Autodesk Inventor part; units mm, degrees
ref_plane "YZ Plane" through (0, 0, 0) normal (1, 0, 0) x (0, 1, 0)
ref_plane "XZ Plane" through (0, 0, 0) normal (0, 1, 0) x (-1, 0, 0)
ref_plane "XY Plane" through (0, 0, 0) normal (0, 0, 1) x (1, 0, 0)
sketch "Sketch1" plane through (0, 0, 0) normal (0, 0, 1) x (1, 0, 0)
  arc A0 (0, 12.7) -> (0, -12.7) centre (0, 0) ccw
  arc A1 (0, 25.4) -> (0, -25.4) centre (0, 0) ccw
  arc A2 (63.5, -12.7) -> (63.5, 12.7) centre (63.5, 0) ccw
  arc A3 (63.5, -25.4) -> (63.5, 25.4) centre (63.5, 0) ccw
  line L0 (0, 12.7) -> (63.5, 12.7)
  line L1 (0, -12.7) -> (63.5, -12.7)
  line L2 (0, 25.4) -> (63.5, 25.4)
  line L3 (0, -25.4) -> (63.5, -25.4)
  dimension "d0" = 25.4
  dimension "d1" = 50.8
  dimension "d2" = 25.4
  dimension "d3" = 50.8
  dimension "d4" = 63.5
extrude "Extrusion1" add sketch "Sketch1" along normal blind 12.7
sketch "Sketch2" plane through (0, 0, 12.7) normal (0, 0, 1) x (1, 0, 0)
  line L0 (0, -25.4) -> (63.5, -25.4)
  line L1 (31.75, -25.4) -> (31.75, -12.7)
  line L2 (0, -12.7) -> (63.5, -12.7)
  line L3 (47.625, -12.7) -> (47.625, -25.4)
  line L4 (95.25, -31.75) -> (95.25, -25.4)
  line L5 (15.875, -12.7) -> (15.875, -25.4)
  line L6 (15.875, -12.7) -> (47.625, -12.7)
  line L7 (15.875, -25.4) -> (47.625, -25.4)
  point P0 (0, 0)
  dimension "d8" = 15.875
  dimension "d9" = 15.875
extrude "Extrusion2" cut sketch "Sketch2" against normal blind 12.7
sketch "Sketch4" plane through (0, 25.4, 0) normal (0, 1, 0) x (1, 0, 0)
  line L0 (63.5, 0) -> (0, 0)
  circle A0 centre (31.75, -25.4) radius 6.35
  arc A1 (15.875, -25.4) -> (47.625, -25.4) centre (31.75, -25.4) ccw
  line L1 (15.875, -25.4) -> (15.875, -12.7)
  line L2 (0, -12.7) -> (15.875, -12.7)
  line L3 (47.625, -25.4) -> (47.625, -12.7)
  line L4 (0, -12.7) -> (63.5, -12.7)
  line L5 (31.75, 0) -> (31.75, -12.7)
  dimension "d15" = 12.7
  dimension "d16" = 31.75
  dimension "d17" = 25.4
  dimension "d20" = 0
extrude "Extrusion3" add sketch "Sketch4" against normal blind 12.7
properties part number "HW 2 Part 4"
Geometry: final body of the model. Coordinates: model frame, mm. A direction names the side the tool comes from. Coordinates: 2 decimals unless noted, no trailing zeros. Order: outer loops, then holes, each group sorted by start corner. A loop starts at its lowest first (then second) coordinate and runs counter-clockwise, first axis right, second up. Notation, with made-up numbers: (-23, 43) - (-5, 43) arc R30 cw to (-5, 69) - close; hole circle Ø3 at (59, 47.5). An arc over 180 degrees is marked (long way). Write each question's results on one line, items separated by ' | '.
(1) First-contact query: pin 1 Ø14 at (y, z) = (16.5, 19) entering from -X; pin 2 Ø12.5 at (x, y) = (69.5, 3) entering from +Z; pin 3 Ø6.5 at (y, z) = (-18, 8) entering from +X. Flat tips, straight axial feed; report the tip coordinate or a pass-through.
Values found:
pin 1: stops at x = -21.55 | pin 2: stops at z = 12.7 | pin 3: stops at x = 84.18
(2) Mould query, pull axis Y, two halves, no side actions, for faces 1 (the face through (88.894, 0.559, 6.261)), 2 (the face through (-12.697, -0.279, 6.261)), 3 (the face through (47.625, -19, 6)), 4 (the face through (31, 12.7, 16)). Classes: +Y half, -Y half, draft (parallel to the pull), parting line (faces both ways), or undercut.
Values found:
face 1: parting line | face 2: undercut | face 3: draft | face 4: undercut
(3) Section query C-C, the plane z = 10. Return the cut outline in (x, y) (3 decimals), plus the area to 3 significant figures.
Values found:
outline: (0, -25.4) - (15.875, -25.4) - (15.875, -12.7) - (0, -12.7) arc R12.7 cw to (0, 12.7) - (63.5, 12.7) arc R12.7 cw to (63.5, -12.7) - (47.625, -12.7) - (47.625, -25.4) - (63.5, -25.4) arc R25.4 ccw to (63.5, 25.4) - (0, 25.4) arc R25.4 ccw to start | area: 2,730 mm²
(4) Set-up query: faces 5 (the face through (15.875, -19, 6)), 6 (the face through (47.625, 19, 19)), 7 (the face through (55, -12.7, 6)). Return all of +Z, -Z, +X, -X, +Y, -Y with unobstructed straight access to the full face (end or side cutting, diameter ignored); none if empty.
Values found:
face 5: +Z, -Z, -Y | face 6: +Z, +X, +Y, -Y | face 7: +Z, -Z
(5) Section query D-D, the plane z = 38. Return the cut outline in (x, y), plus the area to 3 significant figures.
Values found:
outline: (22.09, 12.7) - (41.41, 12.7) - (41.41, 25.4) - (22.09, 25.4) - close | area: 245 mm²
(6) Section query B-B, the plane y = 5.5. Return the cut outline in (x, z), plus the area to 3 significant figures.
Values found:
outline: (-24.8, 0) - (-11.45, 0) - (-11.45, 12.7) - (-24.8, 12.7) - close; (74.95, 0) - (88.3, 0) - (88.3, 12.7) - (74.95, 12.7) - close | area: 339 mm²
(7) Section query A-A, the plane x = 31.75. Return the cut outline in (y, z) (3 decimals), plus the area to 3 significant figures.
Values found:
outline: (12.7, 0) - (25.4, 0) - (25.4, 19.05) - (12.7, 19.05) - close; (12.7, 31.75) - (25.4, 31.75) - (25.4, 41.275) - (12.7, 41.275) - close | area: 363 mm²
(8) Line query: line 1 (Y direction, x = 15, z = 4.5); line 2 (Z direction, x = 31.75, y = 21.25) (3 decimals); line 3 (X direction, y = 18.5, z = 25.4) (3 decimals). Output: solid intervals per line, ascending. Write a range as [from, to].
Values found:
line 1: y = [-25.4, -12.7], [12.7, 25.4] | line 2: z = [0, 19.05], [31.75, 41.275] | line 3: x = [15.875, 25.4], [38.1, 47.625]
